```python
from build123d import *

# Parameters (mm, degrees)
SKETCH1_W           = 34.5
SKETCH1_H           = 49.5
BOSS_EXTRUDE1_DEPTH = 5
SKETCH2_R           = 3.2
CUT_EXTRUDE1_DEPTH  = 5
SKETCH3_W           = 6
SKETCH3_H           = 25
BOSS_EXTRUDE2_DEPTH = 5
FILLET1_R           = 10
FILLET2_R           = 5
SKETCH6_W           = 166.1846994
SKETCH6_H           = 49.5
CUT_EXTRUDE3_DEPTH  = 10
BOSS_EXTRUDE3_DEPTH = 5
SKETCH8_R           = 1.65
CUT_EXTRUDE4_DEPTH  = 10


with BuildPart() as part:
    # Sketch1 → Boss-Extrude1 (new body)
    with BuildSketch(Plane(origin=(0, 0, 0), x_dir=(1, 0, 0), z_dir=(0, 1, 0))):
        with Locations((17.25, 24.75)):
            Rectangle(SKETCH1_W, SKETCH1_H)
    extrude(amount=BOSS_EXTRUDE1_DEPTH)

    # Sketch2 → Cut-Extrude1 (cut)
    with BuildSketch(Plane(origin=(0, 5, 0), x_dir=(1, 0, 0), z_dir=(0, 1, 0))):
        with Locations(Location((5, 39.75, 0), (0, 0, 270))):
            Circle(SKETCH2_R)
        with Locations(Location((5, 9.75, 0), (0, 0, 90))):
            Circle(SKETCH2_R)
        with Locations(Location((29.5, 9.75, 0), (0, 0, 270))):
            Circle(SKETCH2_R)
        with Locations(Location((29.5, 39.75, 0), (0, 0, 90))):
            Circle(SKETCH2_R)
    extrude(amount=-CUT_EXTRUDE1_DEPTH, mode=Mode.SUBTRACT)

    # Sketch3 → Boss-Extrude2 (add)
    with BuildSketch(Plane(origin=(0, 5, 0), x_dir=(1, 0, 0), z_dir=(0, 1, 0))):
        Polygon((189.75, 42.25), (34.5, 49.5), (34.5, 41.491281612), (84.094915791, 39.175254948), (84.094915791, 10.324745052), (34.5, 8.008718388), (34.5, 0), (189.75, 7.25), align=None)
        Polygon((171.053500921, 14.385612956), (89.094915791, 10.558239416), (89.094915791, 38.941760584), (171.053500921, 35.114387044), align=None, mode=Mode.SUBTRACT)
        with Locations((181.13, 24.75)):
            Rectangle(SKETCH3_W, SKETCH3_H, mode=Mode.SUBTRACT)
    extrude(amount=-BOSS_EXTRUDE2_DEPTH)

    # Fillet1
    fillet1_edges = [part.edges().sort_by_distance(p)[0] for p in [
        (34.5, 2.5, -8.008718388),
        (84.094915791, 2.5, -10.324745052),
        (84.094915791, 2.5, -39.175254948),
        (34.5, 2.5, -41.491281612),
        (89.094915791, 2.5, -38.941760584),
        (89.094915791, 2.5, -10.558239416),
    ]]
    fillet(fillet1_edges, radius=FILLET1_R)

    # Fillet2
    fillet2_edges = [part.edges().sort_by_distance(p)[0] for p in [
        (171.053500921, 2.5, -35.114387044),
        (171.053500921, 2.5, -14.385612956),
    ]]
    fillet(fillet2_edges, radius=FILLET2_R)

    # Sketch6 → Cut-Extrude3 (cut)
    with BuildSketch(Plane(origin=(0, 5, 0), x_dir=(1, 0, 0), z_dir=(0, 1, 0))):
        with Locations((117.5923497, 24.75)):
            Rectangle(SKETCH6_W, SKETCH6_H)
    extrude(amount=-CUT_EXTRUDE3_DEPTH, mode=Mode.SUBTRACT)

    # Sketch7 → Boss-Extrude3 (add)
    with BuildSketch(Plane(origin=(0, 5, 0), x_dir=(1, 0, 0), z_dir=(0, 1, 0))):
        Polygon((64.5, 27.75), (34.5, 49.5), (34.5, 0), (64.5, 21.75), (74.5, 21.75), (74.5, 27.75), align=None)
        Polygon((60.119572878, 24.75), (39.5, 39.699190336), (39.5, 9.800809664), align=None, mode=Mode.SUBTRACT)
    extrude(amount=-BOSS_EXTRUDE3_DEPTH)

    # Sketch8 → Cut-Extrude4 (cut)
    with BuildSketch(Plane.XY.offset(-21.75)):
        with Locations((69.5, 2.5)):
            Circle(SKETCH8_R)
    extrude(amount=-CUT_EXTRUDE4_DEPTH, mode=Mode.SUBTRACT)


solid = part.part
```
The model under review builds one solid part; all positions refer to its coordinate system, in mm. A direction names the side the tool comes from. Round coordinates to 2 decimals unless told otherwise and drop trailing zeros. Loops run counter-clockwise (first coordinate to the right, second up) from the corner with the lowest first, then second, coordinate; pieces in that order, holes last. Notation, with made-up numbers: (16.5, -23) -> (61.5, -23) arc R25 cw to (61.5, 11) -> close; hole circle Ø8 at (14, -28.5). An arc over 180 degrees is marked (long way). Answer as a JSON object with one key per item and string values. Group by question number.
1) We need section D-D on x = 29.5. Write out the cut boundary in (y, z).
2) We need section A-A on y = 2.5. Write out the cut boundary in (x, z).
3) Mouldability with a two-part tool opening along X and no side actions: class faces 1 (the face through (68, 4, -21.75)), 2 (the face through (49.71, 2.535, -38.473)), 3 (the face through (68.284, 3.615, -24.708)), 4 (the face through (6.226, 2.535, -12.706)) as released by +X, released by -X, zero draft, split by the parting line, or undercut.
4) We need section B-B on x = 69.5. Write out the cut boundary in (y, z).
5) For line 1 (X direction, y = 2.4, z = -9.75); line 2 (X direction, y = 1.4, z = -40); line 3 (X direction, y = 4.75, z = -12.5), list the stretches that pass through material, from the lowest coordinate up. Write a range as [from, to].
6) For pin 1 Ø5 at (x, z) = (5, -9.75) entering from -Y; pin 2 Ø3 at (x, y) = (47, 2) entering from +Z (3 decimals); pin 3 Ø2.5 at (x, y) = (70, 1.5) entering from -Z, all flat-tipped, find the tip position at first contact; note any pin that passes through.
7) We need section C-C on z = -23.5. Write out the cut boundary in (x, y), then the cut area to 3 significant figures.
8) For faces 5 (the face through (71, 4, -27.75)), 6 (the face through (49.29, 2.535, -10.723)), 7 (the face through (49.665, 2.535, -17.171)), list the 3-axis set-ups (+Z, -Z, +X, -X, +Y, -Y) from which the entire face can be reached by the end or side of a thin tool; tool diameter is ignored.
Result set:
{
 "1": {"outline": "(0, -49.5) -> (5, -49.5) -> (5, -42.95) -> (0, -42.95) -> close; (0, -36.55) -> (5, -36.55) -> (5, -12.95) -> (0, -12.95) -> close; (0, -6.55) -> (5, -6.55) -> (5, 0) -> (0, 0) -> close"},
 "2": {"outline": "(0, -49.5) -> (34.5, -49.5) -> (64.5, -27.75) -> (67.85, -27.75) -> (67.85, -21.75) -> (64.5, -21.75) -> (34.5, 0) -> (0, 0) -> close; (71.15, -27.75) -> (74.5, -27.75) -> (74.5, -21.75) -> (71.15, -21.75) -> close; hole circle Ø6.4 at (5, -39.75); hole circle Ø6.4 at (5, -9.75); hole circle Ø6.4 at (29.5, -39.75); hole circle Ø6.4 at (29.5, -9.75); hole (39.5, -39.7) -> (60.12, -24.75) -> (39.5, -9.8) -> close"},
 "3": {"face 1": "zero draft", "face 2": "released by +X", "face 3": "undercut", "face 4": "undercut"},
 "4": {"outline": "(0, -27.75) -> (0.85, -27.75) -> (0.85, -21.75) -> (0, -21.75) -> close; (4.15, -27.75) -> (5, -27.75) -> (5, -21.75) -> (4.15, -21.75) -> close"},
 "5": {"line 1": "[0, 1.8], [8.2, 26.3], [32.7, 47.95]", "line 2": "[0, 1.81], [8.19, 26.31], [32.69, 47.6]", "line 3": "[0, 3.36], [6.64, 27.86], [31.14, 39.5], [43.22, 51.74]"},
 "6": {"pin 1": "through", "pin 2": "z = -7.975", "pin 3": "z = -27.75"},
 "7": {"outline": "(0, 0) -> (39.5, 0) -> (39.5, 5) -> (0, 5) -> close; (58.4, 0) -> (74.5, 0) -> (74.5, 5) -> (58.4, 5) -> close; hole circle Ø3.3 at (69.5, 2.5)", "area": "269 mm²"},
 "8": {"face 5": "-Z, +X, +Y, -Y", "face 6": "+Z, +X, +Y, -Y", "face 7": "+Y, -Y"}
}
